from build123d import *

# Parameters (mm, degrees)
SKETCH1_R           = 24.875
BOSS_EXTRUDE2_DEPTH = 3
SKETCH1_4_W         = 2.5
SKETCH1_4_H         = 13.6
BOSS_EXTRUDE3_DEPTH = 8.46
CUT_EXTRUDE1_DEPTH  = 2.5
SKETCH5_W           = 4.6
SKETCH5_H           = 13.63
BOSS_EXTRUDE4_DEPTH = 4.95
SKETCH9_W           = 2.6
SKETCH9_H           = 11.63
CUT_EXTRUDE2_DEPTH  = 7.95
SKETCH10_R          = 1.5
CUT_EXTRUDE3_DEPTH  = 4.95


with BuildPart() as part:
    # Sketch1 → Boss-Extrude2 (new body)
    with BuildSketch(Plane.XY):
        Circle(SKETCH1_R)
    extrude(amount=-BOSS_EXTRUDE2_DEPTH)

    # Sketch1<4> → Boss-Extrude3 (add)
    with BuildSketch(Plane.XY):
        with Locations((19.005, 0)):
            Rectangle(SKETCH1_4_W, SKETCH1_4_H)
    extrude(amount=BOSS_EXTRUDE3_DEPTH)

    # Sketch4 → Cut-Extrude1 (cut)
    with BuildSketch(Plane(origin=(20.255, 0, 0), x_dir=(0, 0, -1), z_dir=(1, 0, 0))):
        with BuildLine():
            ThreePointArc((-0.931303911, -0.65), (-3.48591682, 0), (-0.931303911, 0.65))
            Line((-0.931303911, 0.65), (-0.931303911, 5.8))
            Line((-0.931303911, 5.8), (-8.46, 5.8))
            Line((-8.46, 5.8), (-8.46, -5.8))
            Line((-8.46, -5.8), (-0.931303911, -5.8))
            Line((-0.931303911, -5.8), (-0.931303911, -0.65))
        make_face()
    extrude(amount=-CUT_EXTRUDE1_DEPTH, mode=Mode.SUBTRACT)

    # Sketch5 → Boss-Extrude4 (add)
    with BuildSketch(Plane.XY):
        with Locations((-17.96, 0)):
            Rectangle(SKETCH5_W, SKETCH5_H)
    extrude(amount=BOSS_EXTRUDE4_DEPTH)

    # Sketch9 → Cut-Extrude2 (cut)
    with BuildSketch(Plane.XY.offset(4.95)):
        with Locations((-17.96, 0)):
            Rectangle(SKETCH9_W, SKETCH9_H)
    extrude(amount=-CUT_EXTRUDE2_DEPTH, mode=Mode.SUBTRACT)

    # Sketch10 → Cut-Extrude3 (cut)
    with BuildSketch(Plane.XY):
        with Locations((-15.409206931, 12.75144494)):
            Circle(SKETCH10_R)
        with Locations((-15.409206931, -11.899319199)):
            Circle(SKETCH10_R)
    extrude(amount=-CUT_EXTRUDE3_DEPTH, mode=Mode.SUBTRACT)


solid = part.part
Design review of the part built by this model. Coordinates are the model's own, in mm. A direction names the side the tool comes from. Give positions to 0.01 mm unless a question says otherwise; leave off trailing zeros. Write each loop counter-clockwise with the first axis right and the second up, starting at its lowest first coordinate (ties: lowest second). Pieces come first, ordered by that corner, then holes. Notation, with made-up numbers: M 84.5,-24 L 137.5,-24 A15 cw 137.5,-12 Z; hole C 36.5,59.5 d8. An arc over 180 degrees is marked long. Answer as a JSON object with one key per item and string values. Group by question number.
1) We need section D-D (x = 6). Give the boundary of the cut face in (y, z).
2) We need section A-A (z = 7.5). Give the boundary of the cut face in (x, y) (3 decimals), and give its area (3 significant figures).
3) For line 1 along X through (y, z) = (-4, 4.75); line 2 along Y through (x, z) = (19.5, 7); line 3 along X through (y, z) = (-2, -1), list the stretches that pass through material, from the lowest coordinate up.
4) Clearance check with flat-ended pins moving along their axes: pin 1 Ø1 at (y, z) = (4, 4) entering from +X; pin 2 Ø6 at (y, z) = (1, 3.5) entering from +X (3 decimals); pin 3 Ø2.5 at (x, y) = (-15.41, -11.9) entering from +Z; pin 4 Ø6 at (x, z) = (-17, -1) entering from +Y. State where each tip first meets the part, or that it passes through.
5) Mouldability with a two-part tool opening along Y and no side actions: class faces 6 (the face through (-19.26, 0, 1)), 7 (the face through (-18, -6.815, 2)), 8 (the face through (19, 3, 0.931)), 9 (the face through (-15.66, 0, 2)) as released by +Y, released by -Y, zero draft, split by the parting line, or undercut.
6) We need section C-C (z = -0.75). Give the boundary of the cut face in (x, y) (3 decimals).
7) Tool access review of faces 1 (the face through (17.755, 0, 2)), 2 (the face through (-18, 6.815, 2)), 3 (the face through (-20.26, 0, 2)), 4 (the face through (19, -5.8, 5)), 5 (the face through (20.255, 0, 2)): name each direction out of +Z, -Z, +X, -X, +Y, -Y from which nothing blocks a thin tool from reaching the whole face with its end or side.
8) We need section B-B (y = 0). Give the boundary of the cut face in (x, z) (3 decimals).
Answer key:
{
 "1": {"outline": "M -24.14,-3 L 24.14,-3 L 24.14,0 L -24.14,0 Z"},
 "2": {"outline": "M 17.755,-6.8 L 20.255,-6.8 L 20.255,-5.8 L 17.755,-5.8 Z; M 17.755,5.8 L 20.255,5.8 L 20.255,6.8 L 17.755,6.8 Z", "area": "5.00 mm²"},
 "3": {"line 1": "x = -20.26 to -19.26, -16.66 to -15.66", "line 2": "y = -6.8 to -5.8, 5.8 to 6.8", "line 3": "x = -24.79 to -19.26, -16.66 to 24.79"},
 "4": {"pin 1": "stops at x = -15.66", "pin 2": "stops at x = 20.255", "pin 3": "passes through", "pin 4": "stops at y = 20.56"},
 "5": {"face 6": "undercut", "face 7": "released by -Y", "face 8": "undercut", "face 9": "zero draft"},
 "6": {"outline": "C 0,0 d49.75; hole M -19.26,-5.815 L -16.66,-5.815 L -16.66,5.815 L -19.26,5.815 Z; hole C -15.409,-11.899 d3; hole C -15.409,12.751 d3"},
 "7": {"face 1": "+Z, +Y, -Y", "face 2": "+Z, +X, -X, +Y", "face 3": "+Z, -X, +Y, -Y", "face 4": "+Z, +X", "face 5": "+Z, +X, +Y, -Y"},
 "8": {"outline": "M -24.875,-3 L -19.26,-3 L -19.26,4.95 L -20.26,4.95 L -20.26,0 L -24.875,0 Z; M -16.66,-3 L 24.875,-3 L 24.875,0 L 20.255,0 L 20.255,3.486 L 17.755,3.486 L 17.755,0 L -15.66,0 L -15.66,4.95 L -16.66,4.95 Z"}
}
